Design review of the part shown in the three views and the two pictorial views. Dimensions are in mm from the part's minimum x, y and z. A direction names the side the tool comes from. Coordinates: 2 decimals unless noted, no trailing zeros. Loops run counter-clockwise (first coordinate to the right, second up) from the corner with the lowest first, then second, coordinate; pieces in that order, holes last. Notation, with made-up numbers: M 63.5,45 L 72.5,45 A11 ccw 72.5,62 Z; hole C 24,-36.75 d2. An arc over 180 degrees is marked long. Answer as a JSON object with one key per item and string values. Group by question number.
Item 1: Wall thickness on L1, parallel to X at y = 4.75, z = 6.5; L2, parallel to Y at x = 5.25, z = 1.5; L3, parallel to Z at x = 9.5, y = 1: over which ranges is each line inside the solid? List them lowest first. Write a range as from..to.
Item 2: Add section C-C (x = 7.25). State the section outline as (y, z) points, then the cut area to 3 significant figures.
Item 3: Add section B-B (y = 7). State the section outline as (x, z) points.
Item 4: Add section A-A (z = 5.5). State the section outline as (x, y) points, then the cut area to 3 significant figures.
Item 5: Mouldability with a two-part tool opening along X and no side actions: class the marked faces 1, 2, 3 and 4 as +X half, -X half, draft (parallel to the pull), parting line (faces both ways), or undercut.
Item 6: Insertion check: pin 1 (2.5 mm diameter, centred on y = 3.5, z = 8, fed in from -X); pin 2 (0.6 mm diameter, centred on x = 5, z = 10, fed in from +Y); pin 3 (2 mm diameter, centred on x = 13, z = 8, fed in from +Y); pin 4 (4 mm diameter, centred on y = 3.5, z = 7.5, fed in from +X). Each pin has a flat end and moves straight along its axis. Give the tip position at first contact, or say it passes through.
Item 7: Add section D-D (x = 4.5). State the section outline as (y, z) points.
Item 8: Tool access review of the marked faces 5, 6, 7 and 8: name each direction out of +Z, -Z, +X, -X, +Y, -Y from which nothing blocks a thin tool from reaching the whole face with its end or side.
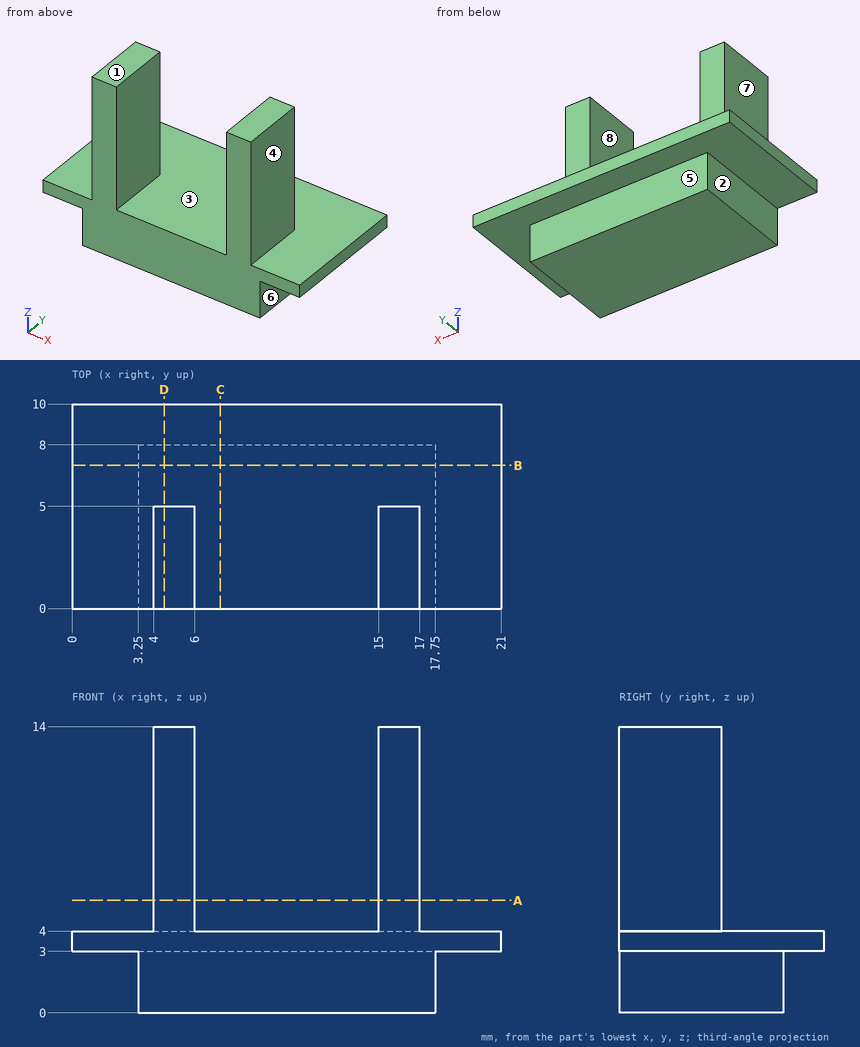
From the geometry:
{
 "1": {"L1": "x = 4..6, 15..17", "L2": "y = 0..8", "L3": "z = 0..4"},
 "2": {"outline": "M 0,0 L 8,0 L 8,3 L 10,3 L 10,4 L 0,4 Z", "area": "34.0 mm²"},
 "3": {"outline": "M 0,3 L 3.25,3 L 3.25,0 L 17.75,0 L 17.75,3 L 21,3 L 21,4 L 0,4 Z"},
 "4": {"outline": "M 4,0 L 6,0 L 6,5 L 4,5 Z; M 15,0 L 17,0 L 17,5 L 15,5 Z", "area": "20.0 mm²"},
 "5": {"face 1": "draft", "face 2": "-X half", "face 3": "undercut", "face 4": "+X half"},
 "6": {"pin 1": "stops at x = 4", "pin 2": "stops at y = 5", "pin 3": "passes through", "pin 4": "stops at x = 17"},
 "7": {"outline": "M 0,0 L 8,0 L 8,3 L 10,3 L 10,4 L 5,4 L 5,14 L 0,14 Z"},
 "8": {"face 5": "-Z, +X, -X, +Y", "face 6": "-Z, +X, +Y, -Y", "face 7": "+Z, -X, +Y, -Y", "face 8": "+Z, +Y, -Y"}
}
